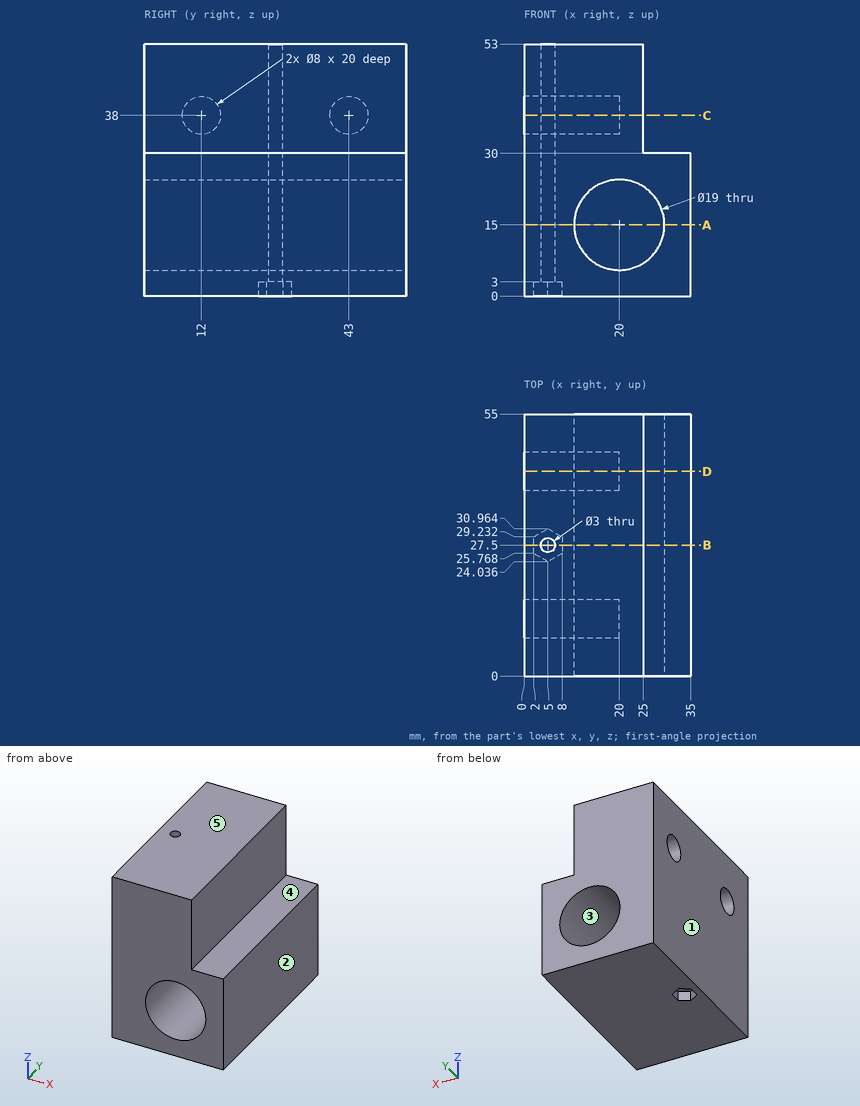
Answer from the drawing. Dimensions are ordinates in mm from the lowest x, y and z of the part. A direction names the side the tool comes from. Coordinates: 2 decimals unless noted, no trailing zeros. Loops run counter-clockwise (first coordinate to the right, second up) from the corner with the lowest first, then second, coordinate; pieces in that order, holes last. Notation, with made-up numbers: (-4.5, -23.5) -> (41.5, -23.5) arc R32 cw to (41.5, 11.5) -> close; hole circle Ø6 at (-27.5, 88.25). An arc over 180 degrees is marked (long way). Return JSON: item names as keys, results as strings.
Item 1: For a pull along X with two mould halves and no side action, classify the marked faces 1, 2 and 3 as +X half, -X half, draft (parallel to the pull), parting line (faces both ways), or undercut.
Answers:
{"face 1": "-X half", "face 2": "+X half", "face 3": "undercut"}
Item 2: Find section D-D (y = 43). Determine the outline of the cut face in (x, z), plus the area to 3 significant figures.
Answers:
{"outline": "(0, 0) -> (35, 0) -> (35, 30) -> (25, 30) -> (25, 53) -> (0, 53) -> (0, 42) -> (20, 42) -> (20, 34) -> (0, 34) -> close; hole circle Ø19 at (20, 15)", "area": "1,180 mm2"}
Item 3: Flat-ended cylindrical pins translate along their axes: P1, Ø6.5, axis at x = 6.5, y = 26.5, coming from the -Z side; P2, Ø1, axis at y = 25, z = 44, coming from the +X side; P3, Ø5, axis at x = 31, y = 34.5, coming from the +Z side; P4, Ø4, axis at x = 5, y = 27.5, coming from the -Z side. Find the tip coordinate at first contact, or state that the pin passes through.
Answers:
{"P1": "stops at z = 0", "P2": "stops at x = 25", "P3": "stops at z = 30", "P4": "stops at z = 3"}
Item 4: For the marked faces 4 and 5, determine the directions among +Z, -Z, +X, -X, +Y, -Y from which every point of the face is accessible in a straight line to the end or side of a thin tool.
Answers:
{"face 4": "+Z, +X, +Y, -Y", "face 5": "+Z, +X, -X, +Y, -Y"}
Item 5: Find section A-A (z = 15). Determine the outline of the cut face in (x, y).
Answers:
{"outline": "(0, 0) -> (10.5, 0) -> (10.5, 55) -> (0, 55) -> close; (29.5, 0) -> (35, 0) -> (35, 55) -> (29.5, 55) -> close; hole circle Ø3 at (5, 27.5)"}
Item 6: Find section C-C (z = 38). Determine the outline of the cut face in (x, y), plus the area to 3 significant figures.
Answers:
{"outline": "(0, 0) -> (25, 0) -> (25, 55) -> (0, 55) -> (0, 47) -> (20, 47) -> (20, 39) -> (0, 39) -> (0, 16) -> (20, 16) -> (20, 8) -> (0, 8) -> close; hole circle Ø3 at (5, 27.5)", "area": "1,050 mm2"}
Item 7: Find section B-B (y = 27.5). Determine the outline of the cut face in (x, z).
Answers:
{"outline": "(0, 0) -> (2, 0) -> (2, 3) -> (3.5, 3) -> (3.5, 53) -> (0, 53) -> close; (6.5, 3) -> (8, 3) -> (8, 0) -> (35, 0) -> (35, 30) -> (25, 30) -> (25, 53) -> (6.5, 53) -> close; hole circle Ø19 at (20, 15)"}
Item 8: Find the intervals of material crossed by probe 1 along Z at (x, y) = (4, 43); probe 2 along X at (y, z) = (27.5, 36); probe 3 along Z at (x, y) = (16, 42), in increasing order.
Answers:
{"probe 1": "z = 0 to 34, 42 to 53", "probe 2": "x = 0 to 3.5, 6.5 to 25", "probe 3": "z = 0 to 6.38, 23.62 to 34.13, 41.87 to 53"}
